Here's how the part is built. I have some questions about the finished solid (model axes, mm). Give positions to 0.01 mm unless a question says otherwise; leave off trailing zeros. Write each loop counter-clockwise with the first axis right and the second up, starting at its lowest first coordinate (ties: lowest second). Pieces come first, ordered by that corner, then holes. Notation, with made-up numbers: (-9.75, 76) - (41.25, 76) arc R13 ccw to (41.25, 81) - close; hole circle Ø7 at (-36, -7.75). An arc over 180 degrees is marked (long way). Write each question's results on one line, items separated by ' | '. Start each with the question number.
Item 1: Will these pins go through, and if not, where does the flat tip stop? P1, Ø9, axis at x = 18, y = 288, coming from the -Z side; P2, Ø9, axis at x = 404.5, y = 479.5, coming from the -Z side.
Item 2: Suppose I cut it at B-B on x = 806. List the corners of the cut face in (y, z) for me, then the cut area to 3 significant figures.
Item 3: Suppose I cut it at A-A on y = 253. List the corners of the cut face in (x, z) for me, then the cut area to 3 significant figures.
Item 4: Please list where these lines run through material, in increasing order: line 1 along X through (y, z) = (93, 77.5); line 2 along Y through (x, z) = (56.5, 80.5); line 3 along Z through (x, y) = (1129.5, 478.5).
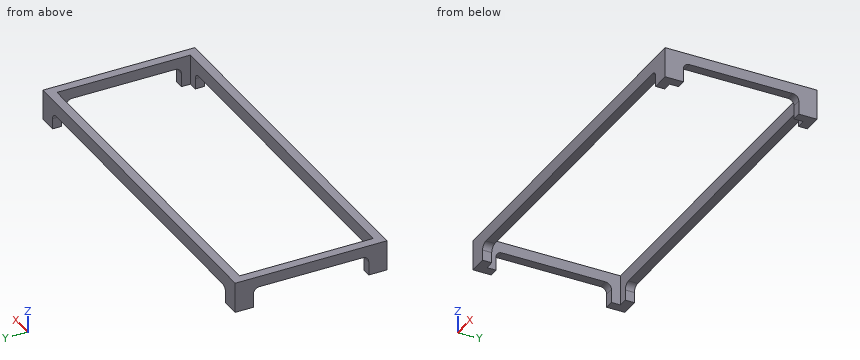
```python
from build123d import *

# Parameters (mm, degrees)
F0_W     = 1200
F0_H     = 500
F0_W_2   = 1140
F0_H_2   = 440
F1_DEPTH = 100
F3_DEPTH = 500.001
F5_DEPTH = 1200.001


with BuildPart() as f1:
    # F0 (on Top) → F1 (new body)
    with BuildSketch(Plane.XY):
        with Locations((600, 250)):
            Rectangle(F0_W, F0_H)
        with Locations((600, 250)):
            Rectangle(F0_W_2, F0_H_2, mode=Mode.SUBTRACT)
    extrude(amount=F1_DEPTH)

    # F2 (on face) → F3 (cut, through all)
    with BuildSketch(Plane.XZ):
        with BuildLine():
            Line((60, 35), (60, 0))
            Line((60, 0), (1140, 0))
            Line((1140, 0), (1140, 35))
            ThreePointArc((1140, 35), (1134.142136, 49.142136), (1120, 55))
            Line((1120, 55), (80, 55))
            ThreePointArc((80, 55), (65.857864, 49.142136), (60, 35))
        make_face()
    extrude(amount=-F3_DEPTH, mode=Mode.SUBTRACT)

    # F4 (on face) → F5 (cut, through all)
    with BuildSketch(Plane(origin=(0, 0, 0), x_dir=(0, -1, 0), z_dir=(-1, 0, 0))):
        with BuildLine():
            Line((-440, 45), (-440, 0))
            Line((-440, 0), (-60, 0))
            Line((-60, 0), (-60, 45))
            ThreePointArc((-60, 45), (-65.857864, 59.142136), (-80, 65))
            Line((-80, 65), (-420, 65))
            ThreePointArc((-420, 65), (-434.142136, 59.142136), (-440, 45))
        make_face()
    extrude(amount=-F5_DEPTH, mode=Mode.SUBTRACT)


solid = f1.part
```
Checked values:
1) P1: stops at z = 65 | P2: stops at z = 55
2) outline: (0, 55) - (30, 55) - (30, 100) - (0, 100) - close; (470, 55) - (500, 55) - (500, 100) - (470, 100) - close | area: 2,700 mm^2
3) outline: (0, 65) - (30, 65) - (30, 100) - (0, 100) - close; (1170, 65) - (1200, 65) - (1200, 100) - (1170, 100) - close | area: 2,100 mm^2
4) line 1: x = 0 to 30, 1170 to 1200 | line 2: y = 0 to 30, 470 to 500 | line 3: z = 52.6 to 100
